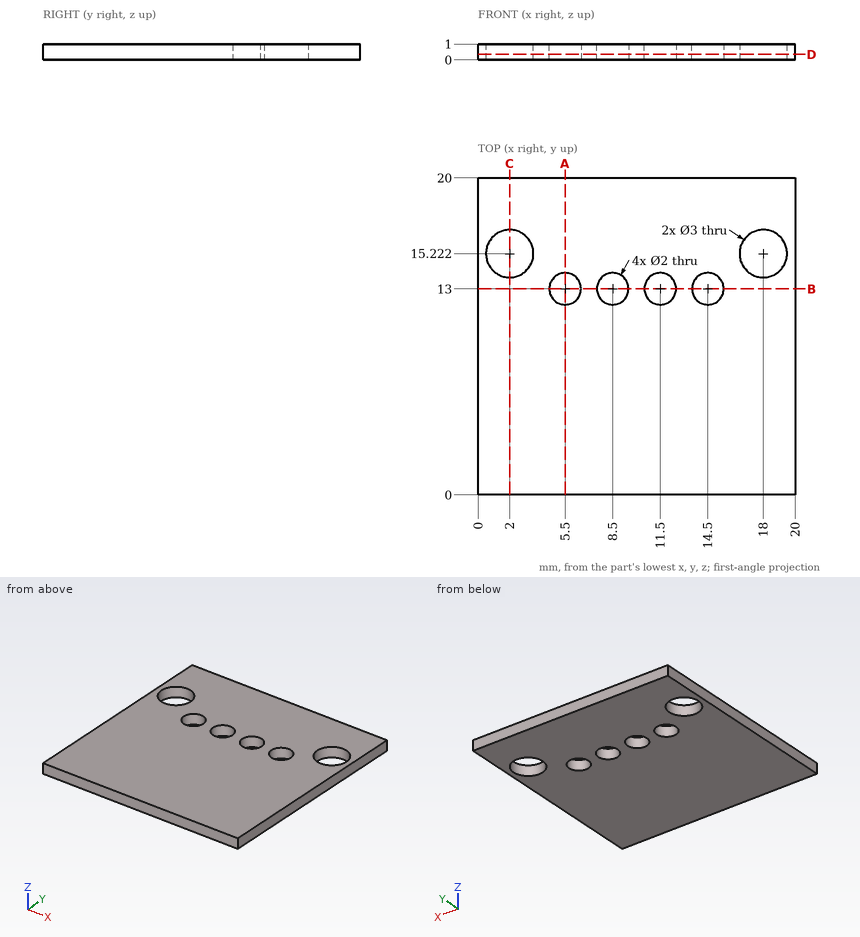
Here's the drawing with two shaded views (mm, measured from the low corner). I have some questions. Give positions to 0.01 mm unless a question says otherwise; leave off trailing zeros. Write each loop counter-clockwise with the first axis right and the second up, starting at its lowest first coordinate (ties: lowest second). Pieces come first, ordered by that corner, then holes. Notation, with made-up numbers: (-3, 53) - (55, 53) arc R20 cw to (55, 63) - close; hole circle Ø11 at (60.5, -35). An arc over 180 degrees is marked (long way). One line per item, written item: value. Start each with the question number.
Item 1: Imagine slicing it at D-D, the plane z = 0.35. List the corners of the cut face in (x, y) for me, and give its area (3 significant figures).
Item 2: Imagine slicing it at A-A, the plane x = 5.5. List the corners of the cut face in (y, z) for me, and give its area (3 significant figures).
Item 3: I'm going to push a flat-ended pin straight in: pin 1 (2.5 mm diameter, centred on x = 2, y = 15.22, fed in from -Z). Where does the tip first touch, or does it pass through?
Item 4: Imagine slicing it at C-C, the plane x = 2. List the corners of the cut face in (y, z) for me.
Item 5: Please list where these lines run through material, in increasing order: line 1 (Y direction, x = 14.5, z = 0.7); line 2 (Y direction, x = 2, z = 0.55). Write a range as from..to.
Item 6: Imagine slicing it at B-B, the plane y = 13. List the corners of the cut face in (x, z) for me.
Geometry says:
1. outline: (0, 0) - (20, 0) - (20, 20) - (0, 20) - close; hole circle Ø3 at (2, 15.22); hole circle Ø2 at (5.5, 13); hole circle Ø2 at (8.5, 13); hole circle Ø2 at (11.5, 13); hole circle Ø2 at (14.5, 13); hole circle Ø3 at (18, 15.22)
1. area: 373 mm^2
2. outline: (0, 0) - (12, 0) - (12, 1) - (0, 1) - close; (14, 0) - (20, 0) - (20, 1) - (14, 1) - close
2. area: 18.0 mm^2
3. pin 1: through
4. outline: (0, 0) - (13.72, 0) - (13.72, 1) - (0, 1) - close; (16.72, 0) - (20, 0) - (20, 1) - (16.72, 1) - close
5. line 1: 0..12, 14..20
5. line 2: 0..13.72, 16.72..20
6. outline: (0, 0) - (4.5, 0) - (4.5, 1) - (0, 1) - close; (6.5, 0) - (7.5, 0) - (7.5, 1) - (6.5, 1) - close; (9.5, 0) - (10.5, 0) - (10.5, 1) - (9.5, 1) - close; (12.5, 0) - (13.5, 0) - (13.5, 1) - (12.5, 1) - close; (15.5, 0) - (20, 0) - (20, 1) - (15.5, 1) - close
